For this review, take the finished solid that the model builds, in its own axes (mm). A direction names the side the tool comes from. Coordinates: 2 decimals unless noted, no trailing zeros. Write each loop counter-clockwise with the first axis right and the second up, starting at its lowest first coordinate (ties: lowest second). Pieces come first, ordered by that corner, then holes. Notation, with made-up numbers: M 89.25,1.25 L 95.25,1.25 A9 cw 95.25,12.25 Z; hole C -22,-18 d5. An arc over 180 degrees is marked long. One line per question, with ' | ' between items.
from build123d import *

# Parameters (mm, degrees)
SKETCH_1_W                 = 20
SKETCH_1_H                 = 10
BASEPLATE_DEPTH            = 1
EDGEFLANGE_STRIP_W         = 8
EDGEFLANGE_STRIP_H         = 1
EDGEFLANGE_STRIP_CUT_DEPTH = 20
EDGEFLANGE_DEPTH           = 20
EDGEFLANGE_START           = 1
EDGEFLANGE_FLAT_DEPTH      = 1


# Sheet-metal steps are written as plain solids
with BuildPart() as part:
    # Sketch 1 → BasePlate (new body)
    with BuildSketch(Plane.XY):
        with Locations((10, 5)):
            Rectangle(SKETCH_1_W, SKETCH_1_H)
    extrude(amount=-BASEPLATE_DEPTH)

    # EdgeFlange strip (across the edge) → EdgeFlange strip cut (cut)
    with BuildSketch(Plane(origin=(20, 10, 0), x_dir=(0, -1, 0), z_dir=(-1, 0, 0))):
        with Locations((-2, -0.5)):
            Rectangle(EDGEFLANGE_STRIP_W, EDGEFLANGE_STRIP_H)
    extrude(amount=EDGEFLANGE_STRIP_CUT_DEPTH, mode=Mode.SUBTRACT)

    # EdgeFlange bend section (across the edge) → EdgeFlange (add)
    with BuildSketch(Plane(origin=(20, 10, 0), x_dir=(0, -1, 0), z_dir=(-1, 0, 0))):
        with BuildLine():
            Line((-1, 2), (0, 2))
            ThreePointArc((0, 2), (0.585786438, 0.585786438), (2, 0))
            Line((2, 0), (2, -1))
            ThreePointArc((2, -1), (-0.121320344, -0.121320344), (-1, 2))
        make_face()
    extrude(amount=EDGEFLANGE_DEPTH)

    # EdgeFlange profile (on flange) → EdgeFlange flat (add)
    with BuildSketch(Plane(origin=(0, 10, 0), x_dir=(-1, 0, 0), z_dir=(0, 1, 0)).offset(EDGEFLANGE_START)):
        Polygon((-20, 10), (-20, 2), (0, 2), (0, 10), (-2, 10), (-18, 10), align=None)
    extrude(amount=-EDGEFLANGE_FLAT_DEPTH)


solid = part.part
1. Machinability: for faces 1 (the flat face through (10, 4, 0)), 2 (the flat face through (9.9, 10.5, 10)), which of the approach directions +Z, -Z, +X, -X, +Y, -Y give a long, thin tool a straight path to every point of the face, cutting with its end or side? Answer none if there is none.
Computed values:
face 1: +Z, +X, -X, -Y | face 2: +Z, +X, -X, +Y, -Y
2. Take a section at A-A on x = 16.75. State the section outline as (y, z) points.
Computed values:
outline: M 0,-1 L 8,-1 A3 ccw 11,2 L 11,10 L 10,10 L 10,2 A2 cw 8,0 L 0,0 Z
3. For line 1 along Z through (x, y) = (12.75, 3); line 2 along Y through (x, z) = (1.5, 8.75); line 3 along Z through (x, y) = (4.75, 8.5), list the stretches that pass through material, from the lowest coordinate up.
Computed values:
line 1: z = -1 to 0 | line 2: y = 10 to 11 | line 3: z = -0.96 to 0.06
4. Take a section at C-C on y = 7.25. State the section outline as (x, z) points, plus the area to 3 significant figures.
Computed values:
outline: M 0,-1 L 20,-1 L 20,0 L 0,0 Z | area: 20.0 mm2
5. Clearance check with flat-ended pins moving along their axes: P1, Ø6.5, axis at x = 7, z = 5, coming from the -Y side; P2, Ø3, axis at y = 2, z = 2, coming from the -X side; P3, Ø4, axis at x = 12, y = 6, coming from the +Z side. State where each tip first meets the part, or that it passes through.
Computed values:
P1: stops at y = 9.98 | P2: passes through | P3: stops at z = 0
6. Take a section at B-B on z = 9. State the section outline as (x, y) points, plus the area to 3 significant figures.
Computed values:
outline: M 0,10 L 20,10 L 20,11 L 0,11 Z | area: 20.0 mm2
